Autodesk Inventor part; units mm, degrees
ref_plane "YZ Plane" through (0, 0, 0) normal (1, 0, 0) x (0, 1, 0)
ref_plane "XZ Plane" through (0, 0, 0) normal (0, 1, 0) x (-1, 0, 0)
ref_plane "XY Plane" through (0, 0, 0) normal (0, 0, 1) x (1, 0, 0)
sketch "Sketch1" plane through (0, 0, 0) normal (0, 1, 0) x (-1, 0, 0)
  arc A0 (-76.2, 0) -> (0, -76.2) centre (0, 0) ccw
  line L0 (-76.2, 0) -> (-31.75, 0)
  line L1 (0, -76.2) -> (0, -31.75)
  arc A1 (-31.75, 0) -> (0, -31.75) centre (0, 0) ccw
  line L2 (0, 0) -> (-35.921, -35.921)
  line L3 (0, 0) -> (50.8, 0) construction
  circle A2 centre (-35.921, -35.921) radius 5.715
  line L4 (-35.921, -35.921) -> (-28.5572, -43.2848)
  line L5 (-35.921, -35.921) -> (-25.507, -35.921) construction
  line L6 (-35.921, -35.921) -> (-43.2848, -28.5572)
  circle A3 centre (-28.5572, -43.2848) radius 1.651
  circle A4 centre (-43.2848, -28.5572) radius 1.651
  dimension "d0" = 152.4
  dimension "d1" = 44.45
  dimension "d2" = 44.45
  dimension "d3" = 50.8
  dimension "d4" = 135
  dimension "d5" = 11.43
  dimension "d6" = 10.414
  dimension "d7" = 45
  dimension "d8" = 10.414
  dimension "d9" = 3.302
  dimension "d10" = 3.302
extrude "Extrusion1" add sketch "Sketch1" along normal blind 3.937
sketch "Sketch4" plane through (0, 3.937, 0) normal (0, 1, 0) x (1, 0, 0)
  circle A0 centre (35.921, 35.921) radius 5.715
  circle A1 centre (43.2848, 28.5572) radius 1.651
  circle A2 centre (28.5572, 43.2848) radius 1.651
  arc A3 (76.2, 0) -> (0, 76.2) centre (0, 0) ccw
  line L0 (0, 76.2) -> (0, 31.75)
  arc A4 (31.75, 0) -> (0, 31.75) centre (0, 0) ccw
  line L1 (31.75, 0) -> (76.2, 0)
  line L2 (5.08, 76.0305) -> (5.08, 31.341)
  line L3 (31.341, 5.08) -> (76.0305, 5.08)
  dimension "d15" = 5.08
  dimension "d16" = 5.08
extrude "Extrusion2" add sketch "Sketch4" along normal blind 7.62 contours L1 A4 L3 A3 | L2 A4 L0 A3
sketch "Sketch5" plane through (31.75, 0, 0) normal (0, 0, 1) x (1, 0, 0)
  line L0 (0, 0) -> (0, 11.557)
  line L1 (0, 7.747) -> (44.3964, 7.747)
  line L2 (0, 11.557) -> (44.45, 11.557)
  circle A0 centre (7.62, 7.747) radius 1.524
  circle A1 centre (36.83, 7.747) radius 1.524
  line L3 (44.45, 0) -> (44.45, 11.557)
  point P0 (-31.75, 0)
  dimension "d19" = 3.81
  dimension "d20" = 3.048
  dimension "d21" = 3.048
  dimension "d22" = 7.62
  dimension "d23" = 7.62
extrude "Extrusion3" cut sketch "Sketch5" against normal through all
sketch "Sketch6" plane through (0, 0, -76.2) normal (-1, 0, 0) x (0, 0, 1)
  line L0 (0.0164, 7.747) -> (43.8758, 7.747)
  line L1 (0, 11.557) -> (44.45, 11.557)
  circle A0 centre (7.6364, 7.747) radius 1.524
  circle A1 centre (36.83, 7.747) radius 1.524
  line L2 (44.45, 0) -> (44.45, 11.557)
  point P0 (76.2, 0)
  dimension "d26" = 3.81
  dimension "d27" = 3.048
  dimension "d28" = 3.048
  dimension "d29" = 7.62
  dimension "d30" = 7.62
extrude "Extrusion4" cut sketch "Sketch6" against normal blind 7.62
sketch "Sketch7" plane through (0, 3.937, 0) normal (0, 1, 0) x (1, 0, 0)
  arc A0 (76.0305, 5.08) -> (5.08, 76.0305) centre (0, 0) ccw
  line L0 (5.08, 31.341) -> (5.08, 76.0305)
  line L1 (76.0305, 5.08) -> (31.341, 5.08)
  arc A1 (66.4812, 5.08) -> (5.08, 66.4812) centre (0, 0) ccw
  dimension "d33" = 133.35
extrude "Extrusion5" add sketch "Sketch7" along normal blind 25.4
properties part number "base_segment"
Here's how the part is built. I have some questions about the finished solid (model axes, mm). A direction names the side the tool comes from. Coordinates: 2 decimals unless noted, no trailing zeros. Order: outer loops, then holes, each group sorted by start corner. A loop starts at its lowest first (then second) coordinate and runs counter-clockwise, first axis right, second up.
Item 1: I'm going to push flat-ended pins straight in: pin 1 Ø4 at (y, z) = (21.5, -48) entering from +X; pin 2 Ø6 at (x, z) = (51, -30) entering from +Y; pin 3 Ø5 at (x, y) = (69, 20.5) entering from +Z; pin 4 Ø3 at (x, z) = (43.28, -28.56) entering from +Y. Where does each tip first touch, or does it pass through?
Response values:
pin 1: stops at x = 60.75
pin 2: stops at y = 3.94
pin 3: stops at z = -5.08
pin 4: passes through
Item 2: If we section it at C-C, the plane z = -22.5: List the corners of the cut face in (x, y) for me.
Response values:
outline: (22.4, 0) - (72.8, 0) - (72.8, 29.34) - (62.76, 29.34) - (62.76, 3.94) - (22.4, 3.94) - close
Item 3: Which directions (+Z, -Z, +X, -X, +Y, -Y) give clear straight access to the entire face, cutting with the end or side of a thin tool? Please do faces 1 (the face through (5.08, 20, -71)), 2 (the face through (29, 3.937, -35)), 3 (the face through (69, 8, -5.08)), 4 (the face through (71, 20, -5.08)), 5 (the face through (2.5, 6.82, -40.58)).
Response values:
face 1: +Z, -Z, -X, +Y
face 2: +Y
face 3: +Z
face 4: +Z, +X, -X, +Y
face 5: -X
Item 4: If we section it at B-B, the plane x = 39.37: List the corners of the cut face in (y, z) for me.
Response values:
outline: (0, -65.24) - (29.34, -65.24) - (29.34, -53.81) - (3.94, -53.81) - (3.94, -40.48) - (0, -40.48) - close; (0, -31.36) - (3.94, -31.36) - (3.94, -5.08) - (6.22, -5.08) - (6.22, 0) - (0, 0) - close; (9.27, -5.08) - (11.56, -5.08) - (11.56, 0) - (9.27, 0) - close
Item 5: If we section it at A-A, the plane z = -33: List the corners of the cut face in (x, y) for me, then the cut area to 3 significant figures.
Response values:
outline: (0, 0) - (31.01, 0) - (31.01, 3.94) - (5.08, 3.94) - (5.08, 11.56) - (0, 11.56) - close; (40.83, 0) - (68.68, 0) - (68.68, 29.34) - (57.94, 29.34) - (57.94, 3.94) - (40.83, 3.94) - close
area: 543 mm2
Item 6: I need wall thicknesses on probe 1 along X at (y, z) = (8.5, -5); probe 2 along Y at (x, z) = (68.58, -3.85); probe 3 along Y at (x, z) = (22.5, -59.5). Which ranges of each line are inside material? Lowest first, please.
Response values:
probe 1: x = 31.35 to 38.05, 40.69 to 67.26, 69.9 to 76.04
probe 2: y = 0 to 6.22, 9.27 to 11.56
probe 3: y = 0 to 3.94
Item 7: Thinking about a two-plate mould opening in Y: for faces 6 (the face through (53, 11.557, -3)), 7 (the face through (28.915, 1.941, -41.673)), 8 (the face through (69.988, 7.163, -2.504)), which applies, pulls with the +Y half, pulls with the -Y half, needs draft (parallel to the pull), parting line crosses it, or undercut?
Response values:
face 6: pulls with the +Y half
face 7: needs draft
face 8: undercut
